Build history of the part. All positions in model axes, mm. Face numbers are marked on the shaded views. Give positions to 0.01 mm unless a question says otherwise; leave off trailing zeros. One line per question, with ' | ' between items. Start each with the question number.
(1) Drill centre lines: L1, parallel to X at y = 19, z = 0.25; L2, parallel to Z at x = -21, y = 36.5; L3, parallel to Y at x = -29.5, z = 3.5. Where is each one in solid material? Low to high. Write a range as from..to.
(2) Pin check, flat tips, straight feed: pin 1 Ø4 at (y, z) = (28.5, -3.5) entering from -X; pin 2 Ø6 at (y, z) = (9, -3.5) entering from +X; pin 3 Ø1.6 at (y, z) = (0.5, 0) entering from -X. Stop position of each tip, or through.
(3) Cut at A-A (z = -0.5). Give the number of separate pieces and of enclosed holes in the cut face, then the cut area to 3 significant figures.
(4) Pull direction X, two halves, no side cores. Call the marked faces 1, 2 and 3: +X half, -X half, draft (parallel to the pull), parting line (faces both ways), or undercut.
from build123d import *

# Parameters (mm, degrees)
CUT_EXTRUDE1_REACH      = 73.67
CUT_EXTRUDE1_END_RADIUS = 11.509727536


with BuildPart() as part:
    # Sweep3: sweep along a path in swept profile
    with BuildLine(Plane.XY) as sweep3_path:
        Line((27, 0), (32, 0))
        ThreePointArc((32, 0), (33.414213562, 0.585786438), (34, 2))
        Line((34, 2), (34, 22.971251236))
        ThreePointArc((34, 22.971251236), (33.633140648, 24.851146908), (32.586396904, 26.455179657))
        Line((32.586396904, 26.455179657), (3.586396904, 56.308120834))
        ThreePointArc((3.586396904, 56.308120834), (0, 57.824192412), (-3.586396904, 56.308120834))
        Line((-3.586396904, 56.308120834), (-32.586396904, 26.455179657))
        ThreePointArc((-32.586396904, 26.455179657), (-33.633140648, 24.851146908), (-34, 22.971251236))
        Line((-34, 22.971251236), (-34, 2))
        ThreePointArc((-34, 2), (-33.414213562, 0.585786438), (-32, 0))
        Line((-32, 0), (-27, 0))
    # guide line → Sweep3 (sweep)
    with BuildSketch(Plane(origin=(27, 0, 0), x_dir=(0, 0, -1), z_dir=(1, 0, 0))):
        with BuildLine():
            ThreePointArc((-5.010561558, 0.547286439), (0, -0.5), (5.010561558, 0.547286439))
            ThreePointArc((5.010561558, 0.547286439), (5.268436061, 1.20569417), (4.610028329, 1.463568673))
            ThreePointArc((4.610028329, 1.463568673), (0, 0.5), (-4.610028329, 1.463568673))
            ThreePointArc((-4.610028329, 1.463568673), (-5.268436061, 1.20569417), (-5.010561558, 0.547286439))
        make_face()
    sweep(path=sweep3_path.line)

    # Cut-Extrude1: up to this cylinder (the profile starts outside it)
    cut_extrude1_end = Plane(origin=(-10.201880326, 32.262165574, 0), z_dir=(-0.6967856842632488, -0.717279380859227, 0)) * Cylinder(CUT_EXTRUDE1_END_RADIUS, 171.359455073, mode=Mode.PRIVATE)
    # Sketch66 → Cut-Extrude1 (cut, up to the surface)
    with BuildSketch(Plane(origin=(-29.616848042, 28.770652384, 7.029029048), x_dir=(-0.6967856842632488, -0.717279380859227, 0), z_dir=(-0.7071067811865512, 0.6869037302955067, 0.16781914463526715)), mode=Mode.PRIVATE) as cut_extrude1_sk1:
        with BuildLine():
            Line((-30.115399458, -4.545589627), (-1.94952466, -4.545589627))
            ThreePointArc((-1.94952466, -4.545589627), (0.55579574, -7.050910027), (-1.94952466, -9.556230427))
            Line((-1.94952466, -9.556230427), (-30.115399458, -9.556230427))
            ThreePointArc((-30.115399458, -9.556230427), (-32.620719857, -7.050910027), (-30.115399458, -4.545589627))
        make_face()
    cut_extrude1_tool1 = extrude(cut_extrude1_sk1.sketch, amount=-CUT_EXTRUDE1_REACH, mode=Mode.PRIVATE) - cut_extrude1_end
    cut_extrude1 = cut_extrude1_tool1.solids().sort_by_distance((-19.294399, 41.094898, 0.078116))[0]
    add(cut_extrude1, mode=Mode.SUBTRACT)

    # Mirror1: Cut-Extrude1 across plane
    add(cut_extrude1.mirror(Plane(origin=(0, 0, 0), x_dir=(0, 0, 1), z_dir=(1, 0, 0))), mode=Mode.SUBTRACT)


solid = part.part
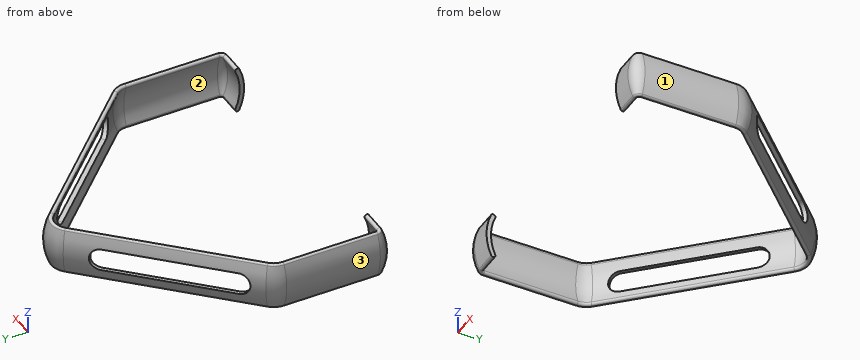
Result set:
1) L1: x = -34.5..-33.5, 33.5..34.5 | L2: z = -5.21..-4.25, 4.25..5.21 | L3: y = 0..1.05, 28.13..29.63
2) pin 1: stops at x = -32.68 | pin 2: stops at x = 34.49 | pin 3: stops at x = -34.4
3) separate pieces: 3 | enclosed holes: 0 | area: 91.0 mm2
4) face 1: +X half | face 2: undercut | face 3: -X half
